from build123d import *

# Parameters (mm, degrees)
ESBO_O1_W                = 35
ESBO_O1_H                = 9.5
ESBO_O1_W_2              = 105
ESBO_O1_H_2              = 20
BASE_DEPTH               = 1.2
ESBO_O2_W                = 32.6
ESBO_O2_H                = 15.6
SUPORTE_1_DEPTH          = 17
ESBO_O3_W                = 23.6
ESBO_O3_H                = 12.6
CORTE_EXTRUS_O1_DEPTH    = 19.5
ESBO_O4_W                = 16.6
ESBO_O4_H                = 17.237895569
CORTE_EXTRUS_O2_DEPTH    = 19.5
ESBO_O5_W                = 11.4
ESBO_O5_H                = 14
CORTE_EXTRUS_O3_DEPTH    = 36.5
ESBO_O6_R                = 0.75
CORTE_EXTRUS_O4_DEPTH    = 7.5
ESBO_O7_W                = 35
ESBO_O7_H                = 8
RESSALTO_EXTRUS_O3_DEPTH = 35.24
ESBO_O9_W                = 23
ESBO_O9_H                = 25.2
CORTE_EXTRUS_O5_DEPTH    = 22.5
ESBO_O10_R               = 0.75
CORTE_EXTRUS_O6_DEPTH    = 22.5
CHANFRO1_SIZE            = 2
CHANFRO2_SIZE            = 2
FILETE1_R                = 1
FILETE2_R                = 1
FILETE3_R                = 1
FILETE4_R                = 1
FILETE5_R                = 1
FILETE6_R                = 1
FILETE7_R                = 1
FILETE8_R                = 1
FILETE9_RADIUS           = 0.75
FILETE9_LENGTH           = 14
FILETE10_RADIUS          = 0.75
FILETE10_LENGTH          = 14
FILETE11_RADIUS          = 0.75
FILETE11_LENGTH          = 14
FILETE12_RADIUS          = 0.75
FILETE12_LENGTH          = 14
FILETE13_R               = 1
FILETE14_R               = 1
FILETE15_R               = 1
FILETE16_R               = 1
FILETE17_R               = 4
FILETE18_R               = 4
FILETE19_R               = 4
FILETE20_R               = 4


with BuildPart() as part:
    # Esboço1 → Base (new body)
    with BuildSketch(Plane(origin=(0, 0, 0), x_dir=(1, 0, 0), z_dir=(0, 1, 0))):
        with Locations((35, 14.75)):
            Rectangle(ESBO_O1_W, ESBO_O1_H)
        Rectangle(ESBO_O1_W_2, ESBO_O1_H_2)
    extrude(amount=BASE_DEPTH)

    # Esboço2 → Suporte 1 (add)
    with BuildSketch(Plane(origin=(0, 1.2, 0), x_dir=(1, 0, 0), z_dir=(0, 1, 0))):
        with Locations((-32.7, 0)):
            Rectangle(ESBO_O2_W, ESBO_O2_H)
    extrude(amount=SUPORTE_1_DEPTH)

    # Esboço3 → Corte-extrusão1 (cut)
    with BuildSketch(Plane(origin=(0, 18.2, 0), x_dir=(1, 0, 0), z_dir=(0, 1, 0))):
        with Locations((-32.7, 0)):
            Rectangle(ESBO_O3_W, ESBO_O3_H)
    extrude(amount=-CORTE_EXTRUS_O1_DEPTH, mode=Mode.SUBTRACT)

    # Esboço4 → Corte-extrusão2 (cut)
    with BuildSketch(Plane.XY.offset(7.8)):
        with Locations((-32.7, 12.818947785)):
            Rectangle(ESBO_O4_W, ESBO_O4_H)
    extrude(amount=-CORTE_EXTRUS_O2_DEPTH, mode=Mode.SUBTRACT)

    # Esboço5 → Corte-extrusão3 (cut)
    with BuildSketch(Plane(origin=(-16.4, 0, 0), x_dir=(0, 0, -1), z_dir=(1, 0, 0))):
        with Locations((0, 8.2)):
            Rectangle(ESBO_O5_W, ESBO_O5_H)
    extrude(amount=-CORTE_EXTRUS_O3_DEPTH, mode=Mode.SUBTRACT)

    # Esboço6 → Corte-extrusão4 (cut)
    with BuildSketch(Plane(origin=(0, 18.2, 0), x_dir=(1, 0, 0), z_dir=(0, 1, 0))):
        with Locations(Location((-47, 0, 0), (0, 0, 270))):
            Circle(ESBO_O6_R)
        with Locations(Location((-18.4, 0, 0), (0, 0, 270))):
            Circle(ESBO_O6_R)
    extrude(amount=-CORTE_EXTRUS_O4_DEPTH, mode=Mode.SUBTRACT)

    # Esboço7 → Ressalto-extrusão3 (add)
    with BuildSketch(Plane(origin=(0, 1.2, 0), x_dir=(1, 0, 0), z_dir=(0, 1, 0))):
        with Locations((35, 15.5)):
            Rectangle(ESBO_O7_W, ESBO_O7_H)
    extrude(amount=RESSALTO_EXTRUS_O3_DEPTH)

    # Esboço9 → Corte-extrusão5 (cut)
    with BuildSketch(Plane.XY.offset(-11.5)):
        with Locations((35, 36.44)):
            Rectangle(ESBO_O9_W, ESBO_O9_H)
    extrude(amount=-CORTE_EXTRUS_O5_DEPTH, mode=Mode.SUBTRACT)

    # Esboço10 → Corte-extrusão6 (cut)
    with BuildSketch(Plane.XY.offset(-11.5)):
        with Locations((21, 30.14)):
            Circle(ESBO_O10_R)
        with Locations((49, 30.14)):
            Circle(ESBO_O10_R)
    extrude(amount=-CORTE_EXTRUS_O6_DEPTH, mode=Mode.SUBTRACT)

    # Chanfro1
    chanfro1_edges = [part.edges().sort_by_distance(p)[0] for p in [
        (-32.7, 1.2, 7.8),
    ]]
    chamfer(chanfro1_edges, length=CHANFRO1_SIZE)

    # Chanfro2
    chanfro2_edges = [part.edges().sort_by_distance(p)[0] for p in [
        (-32.7, 1.2, -7.8),
    ]]
    chamfer(chanfro2_edges, length=CHANFRO2_SIZE)

    # Filete1
    filete1_edges = [part.edges().sort_by_distance(p)[0] for p in [
        (52.5, 18.22, -19.5),
    ]]
    fillet(filete1_edges, radius=FILETE1_R)

    # Filete2
    filete2_edges = [part.edges().sort_by_distance(p)[0] for p in [
        (17.5, 18.22, -19.5),
    ]]
    fillet(filete2_edges, radius=FILETE2_R)

    # Filete3
    filete3_edges = [part.edges().sort_by_distance(p)[0] for p in [
        (23.5, 30.14, -19.5),
    ]]
    fillet(filete3_edges, radius=FILETE3_R)

    # Filete4
    filete4_edges = [part.edges().sort_by_distance(p)[0] for p in [
        (46.5, 30.14, -19.5),
    ]]
    fillet(filete4_edges, radius=FILETE4_R)

    # Filete5
    filete5_edges = [part.edges().sort_by_distance(p)[0] for p in [
        (52.5, 18.82, -11.5),
    ]]
    fillet(filete5_edges, radius=FILETE5_R)

    # Filete6
    filete6_edges = [part.edges().sort_by_distance(p)[0] for p in [
        (17.5, 18.82, -11.5),
    ]]
    fillet(filete6_edges, radius=FILETE6_R)

    # Filete7
    filete7_edges = [part.edges().sort_by_distance(p)[0] for p in [
        (46.5, 30.14, -11.5),
    ]]
    fillet(filete7_edges, radius=FILETE7_R)

    # Filete8
    filete8_edges = [part.edges().sort_by_distance(p)[0] for p in [
        (23.5, 30.14, -11.5),
    ]]
    fillet(filete8_edges, radius=FILETE8_R)

    # Filete9: full round fillet: the end face becomes a half cylinder, R = half its width
    filete9_face = Plane((-41, 11.2, 7.05), x_dir=(0, -1, 0), z_dir=(1, 0, 0))  # on the end face: x along it, z out of the body
    filete9_slab = filete9_face.offset(-FILETE9_RADIUS / 2) * Box(FILETE9_LENGTH, 2 * FILETE9_RADIUS, FILETE9_RADIUS, mode=Mode.PRIVATE)  # the body's end, R deep
    filete9_round = Plane((-41.75, 11.2, 7.05), x_dir=(1, 0, 0), z_dir=(0, -1, 0)) * Cylinder(FILETE9_RADIUS, FILETE9_LENGTH, mode=Mode.PRIVATE)  # its axis R under the face
    add(filete9_slab - filete9_round, mode=Mode.SUBTRACT)

    # Filete10: full round fillet: the end face becomes a half cylinder, R = half its width
    filete10_face = Plane((-41, 11.2, -7.05), x_dir=(0, -1, 0), z_dir=(1, 0, 0))  # on the end face: x along it, z out of the body
    filete10_slab = filete10_face.offset(-FILETE10_RADIUS / 2) * Box(FILETE10_LENGTH, 2 * FILETE10_RADIUS, FILETE10_RADIUS, mode=Mode.PRIVATE)  # the body's end, R deep
    filete10_round = Plane((-41.75, 11.2, -7.05), x_dir=(1, 0, 0), z_dir=(0, -1, 0)) * Cylinder(FILETE10_RADIUS, FILETE10_LENGTH, mode=Mode.PRIVATE)  # its axis R under the face
    add(filete10_slab - filete10_round, mode=Mode.SUBTRACT)

    # Filete11: full round fillet: the end face becomes a half cylinder, R = half its width
    filete11_face = Plane((-24.4, 11.2, 7.05), x_dir=(0, 1, 0), z_dir=(-1, 0, 0))  # on the end face: x along it, z out of the body
    filete11_slab = filete11_face.offset(-FILETE11_RADIUS / 2) * Box(FILETE11_LENGTH, 2 * FILETE11_RADIUS, FILETE11_RADIUS, mode=Mode.PRIVATE)  # the body's end, R deep
    filete11_round = Plane((-23.65, 11.2, 7.05), x_dir=(-1, 0, 0), z_dir=(0, 1, 0)) * Cylinder(FILETE11_RADIUS, FILETE11_LENGTH, mode=Mode.PRIVATE)  # its axis R under the face
    add(filete11_slab - filete11_round, mode=Mode.SUBTRACT)

    # Filete12: full round fillet: the end face becomes a half cylinder, R = half its width
    filete12_face = Plane((-24.4, 11.2, -7.05), x_dir=(0, 1, 0), z_dir=(-1, 0, 0))  # on the end face: x along it, z out of the body
    filete12_slab = filete12_face.offset(-FILETE12_RADIUS / 2) * Box(FILETE12_LENGTH, 2 * FILETE12_RADIUS, FILETE12_RADIUS, mode=Mode.PRIVATE)  # the body's end, R deep
    filete12_round = Plane((-23.65, 11.2, -7.05), x_dir=(-1, 0, 0), z_dir=(0, 1, 0)) * Cylinder(FILETE12_RADIUS, FILETE12_LENGTH, mode=Mode.PRIVATE)  # its axis R under the face
    add(filete12_slab - filete12_round, mode=Mode.SUBTRACT)

    # Filete13
    filete13_edges = [part.edges().sort_by_distance(p)[0] for p in [
        (-49, 10.7, -7.8),
    ]]
    fillet(filete13_edges, radius=FILETE13_R)

    # Filete14
    filete14_edges = [part.edges().sort_by_distance(p)[0] for p in [
        (-49, 10.7, 7.8),
    ]]
    fillet(filete14_edges, radius=FILETE14_R)

    # Filete15
    filete15_edges = [part.edges().sort_by_distance(p)[0] for p in [
        (-16.4, 10.7, 7.8),
    ]]
    fillet(filete15_edges, radius=FILETE15_R)

    # Filete16
    filete16_edges = [part.edges().sort_by_distance(p)[0] for p in [
        (-16.4, 10.7, -7.8),
    ]]
    fillet(filete16_edges, radius=FILETE16_R)

    # Filete17
    filete17_edges = [part.edges().sort_by_distance(p)[0] for p in [
        (-52.5, 0.6, 10),
    ]]
    fillet(filete17_edges, radius=FILETE17_R)

    # Filete18
    filete18_edges = [part.edges().sort_by_distance(p)[0] for p in [
        (-52.5, 0.6, -10),
    ]]
    fillet(filete18_edges, radius=FILETE18_R)

    # Filete19
    filete19_edges = [part.edges().sort_by_distance(p)[0] for p in [
        (52.5, 0.6, 10),
    ]]
    fillet(filete19_edges, radius=FILETE19_R)

    # Filete20
    # the kernel refuses this fillet: 4 mm, written as the material it adds along each edge
    with BuildSketch(Plane(origin=(17.5, 0, -10), x_dir=(-1, 0, 0), z_dir=(0, 1, 0))) as filete20_piece_1:
        with BuildLine():
            CenterArc((FILETE20_R, -FILETE20_R), FILETE20_R, 90, 90)
            Line((0, -FILETE20_R), (0, 0))
            Line((0, 0), (FILETE20_R, 0))
        make_face()
    extrude(amount=1.2)


solid = part.part
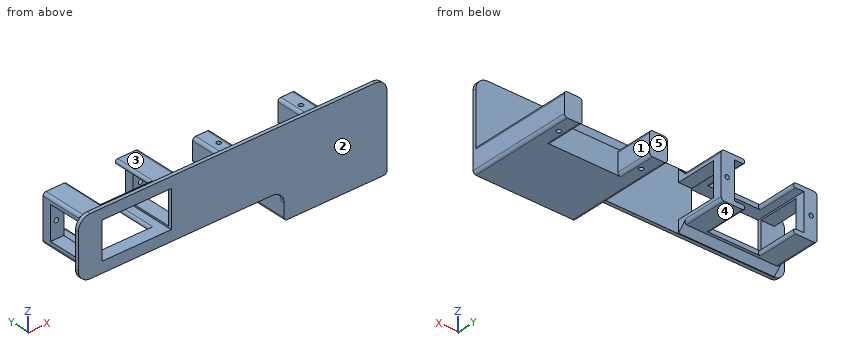
Here's how the part is built. I have some questions about the finished solid (model axes, mm). Face numbers are marked on the shaded views. A direction names the side the tool comes from. Round coordinates to 2 decimals unless told otherwise and drop trailing zeros. Loops run counter-clockwise (first coordinate to the right, second up) from the corner with the lowest first, then second, coordinate; pieces in that order, holes last. Notation, with made-up numbers: (-39, 61.25) - (9, 61.25) arc R26 ccw to (9, 86.25) - close; hole circle Ø2 at (69, 19). An arc over 180 degrees is marked (long way). One line per question, with ' | ' between items. Start each with the question number.
Q1. I want a section at C-C (x = 43). Write out the boundary of the cut face in (y, z), then the cut area to 3 significant figures.
Q2. I want a section at A-A (z = 4.75). Write out the boundary of the cut face in (x, y).
Q3. Will these pins go through, and if not, where does the flat tip stop? pin 1 (1.7 mm diameter, centred on x = 21, y = 30.14, fed in from +Z); pin 2 (1.4 mm diameter, centred on x = 49, y = 30.14, fed in from +Z); pin 3 (1.6 mm diameter, centred on x = -28.5, z = -7, fed in from +Y); pin 4 (6 mm diameter, centred on x = -24, y = 5, fed in from -Z).
Q4. Please list where these lines run through material, in increasing order: line 1 (X direction, y = 16.95, z = 0); line 2 (Y direction, x = 49, z = -15); line 3 (Z direction, x = -47, y = 16). Write a range as [from, to].
Q5. For the marked faces 1 and 2, which set-ups out of +Z, -Z, +X, -X, +Y, -Y let a thin tool reach every point of the face, with its end or its side?
Q6. We'd pull the mould along Z, two halves only. Please class the marked faces 3, 4 and 5: +Z half, -Z half, draft (parallel to the pull), parting line (faces both ways), or undercut.
Q7. I want a section at D-D (x = -14). Write out the boundary of the cut face in (y, z), then the cut area to 3 significant figures.
Q8. I want a section at B-B (y = 27). Write out the boundary of the cut face in (x, z).
Response values:
1) outline: (0, -19.5) - (23.84, -19.5) - (23.84, -11.5) - (1.2, -11.5) - (1.2, 10) - (0, 10) - close | area: 217 mm²
2) outline: (-52.5, 0) - (-44.5, 0) - (-44.5, 1.2) - (-52.5, 1.2) - close; (-49, 15.2) - (-44.5, 15.2) - (-44.5, 18.2) - (-49, 18.2) - close; (-20.9, 0) - (52.5, 0) - (52.5, 1.2) - (-20.9, 1.2) - close; (-20.9, 15.2) - (-16.4, 15.2) - (-16.4, 18.2) - (-20.9, 18.2) - close
3) pin 1: stops at z = -11.5 | pin 2: passes through | pin 3: stops at y = 4.2 | pin 4: stops at z = -9
4) line 1: x = [-49, -47.75], [-46.25, -44.5], [-20.9, -19.15], [-17.65, -16.4] | line 2: y = [0, 29.39], [30.89, 36.44] | line 3: z = [-7.8, -0.75], [0.75, 7.8]
5) face 1: +Z, -Z, +Y | face 2: +Z, -Z, +X, -X, -Y
6) face 3: +Z half | face 4: -Z half | face 5: draft
7) outline: (0, -10) - (1.2, -10) - (1.2, 10) - (0, 10) - close | area: 24.0 mm²
8) outline: (17.5, -18.5) arc R1 ccw to (18.5, -19.5) - (22.5, -19.5) arc R1 ccw to (23.5, -18.5) - (23.5, -12.5) arc R1 ccw to (22.5, -11.5) - (18.5, -11.5) arc R1 ccw to (17.5, -12.5) - close; (46.5, -18.5) arc R1 ccw to (47.5, -19.5) - (51.5, -19.5) arc R1 ccw to (52.5, -18.5) - (52.5, -12.5) arc R1 ccw to (51.5, -11.5) - (47.5, -11.5) arc R1 ccw to (46.5, -12.5) - close
